Design review of the part built by this model. Coordinates are the model's own, in mm. A direction names the side the tool comes from. Give positions to 0.01 mm unless a question says otherwise; leave off trailing zeros. Order: outer loops, then holes, each group sorted by start corner. A loop starts at its lowest first (then second) coordinate and runs counter-clockwise, first axis right, second up. Notation, with made-up numbers: (87, -2) -> (139, -2) arc R27 ccw to (139, 23) -> close; hole circle Ø6 at (71.25, 10.25). An arc over 180 degrees is marked (long way). One line per item, written item: value. Start each with the question number.
1) Consider section B-B (x = 7.5). State the section outline as (y, z) points.
2) Consider section C-C (y = 30). State the section outline as (x, z) points, plus the area to 3 significant figures.
3) The part is to be moulded in two halves that separate along Y. For faces 5 (the face through (43.196, 2.465, -90.789)), 6 (the face through (6.892, 20.099, -20.006)), 7 (the face through (10, 0, -69)), 8 (the face through (2.81, 31.487, 0.195)), say which applies: released by +Y, released by -Y, zero draft, split by the parting line, or undercut.
4) Wall thickness on line 1 along X through (y, z) = (3, -60); line 2 along Y through (x, z) = (26, -57); line 3 along Y through (x, z) = (17.45, 0): over which ranges is each line inside the solid? List them lowest first. Write a range as from..to.
5) Consider section A-A (z = 0). State the section outline as (x, y) points, plus the area to 3 significant figures.
6) Consider section D-D (z = -34). State the section outline as (x, y) points.
7) Tool access review of faces 1 (the face through (45, 2, -85)), 2 (the face through (13.042, 20.065, -20.073)), 3 (the face through (43.289, 2.465, -79.304)), 4 (the face through (13.196, 2.465, -90.789)): name each direction out of +Z, -Z, +X, -X, +Y, -Y from which nothing blocks a thin tool from reaching the whole face with its end or side.
8) For pin 1 (1.5 mm diameter, centred on y = 2.5, z = -71, fed in from +X); pin 2 (6 mm diameter, centred on y = 9.5, z = -34, fed in from +X); pin 3 (4 mm diameter, centred on y = 30, z = 0, fed in from -X), all flat-tipped, find the tip position at first contact; note any pin that passes through.
from build123d import *

# Parameters (mm, degrees)
SKETCH1_R           = 1.5
BOSS_EXTRUDE1_DEPTH = 20
SKETCH2_W           = 8.6
SKETCH2_H           = 36.312939462
CUT_EXTRUDE1_DEPTH  = 20
FILLET2_R           = 5
SKETCH3_R           = 3.05
BOSS_EXTRUDE3_DEPTH = 5
FILLET3_R           = 5
FILLET4_R           = 5


with BuildPart() as part:
    # Sketch1 → Boss-Extrude1 (new body)
    with BuildSketch(Plane(origin=(0, 0, 0), x_dir=(0, 0, -1), z_dir=(1, 0, 0))):
        with BuildLine():
            Line((2.906888371, 35.813776741), (74.534441854, 0))
            Line((74.534441854, 0), (45.465558146, 0))
            Line((45.465558146, 0), (-2.906888371, 24.186223259))
            ThreePointArc((-2.906888371, 24.186223259), (-5.813776741, 32.906888371), (2.906888371, 35.813776741))
        make_face()
        with Locations((0, 30)):
            Circle(SKETCH1_R, mode=Mode.SUBTRACT)
    extrude(amount=BOSS_EXTRUDE1_DEPTH)

    # Sketch2 → Cut-Extrude1 (cut)
    with BuildSketch(Plane(origin=(0, 29.813776741, -14.906888371), x_dir=(1, 0, 0), z_dir=(0, 0.894427190999916, -0.4472135954999577))):
        with Locations((10, -7.492276671)):
            Rectangle(SKETCH2_W, SKETCH2_H)
    extrude(amount=-CUT_EXTRUDE1_DEPTH, mode=Mode.SUBTRACT)

    # Fillet2
    # the kernel refuses this fillet: 5 mm, written as the material it adds along each edge
    with BuildSketch(Plane(origin=(5.7, 25.04460462, -24.445232613), x_dir=(1, 0, 0), z_dir=(0, -0.894427190999916, 0.4472135954999577)), Plane(origin=(14.3, 25.04460462, -24.445232613), x_dir=(0, 0.44721359549995776, 0.894427190999916), z_dir=(0, -0.894427190999916, 0.4472135954999577))) as fillet2_piece_1:
        with BuildLine():
            CenterArc((FILLET2_R, FILLET2_R), FILLET2_R, 180, 90)
            Line((0, FILLET2_R), (0, 0))
            Line((0, 0), (FILLET2_R, 0))
        make_face()
    extrude(amount=13)

    # Sketch3 → Boss-Extrude3 (add)
    with BuildSketch(Plane.XZ):
        with BuildLine():
            Line((-19, -92.5), (-16, -92.5))
            ThreePointArc((-16, -92.5), (-11.757359313, -90.742640687), (-10, -86.5))
            Line((-10, -86.5), (-10, -85))
            Line((-10, -85), (0, -85))
            Line((0, -85), (0, -86.5))
            ThreePointArc((0, -86.5), (1.757359313, -90.742640687), (6, -92.5))
            Line((6, -92.5), (9, -92.5))
            ThreePointArc((9, -92.5), (13.242640687, -90.742640687), (15, -86.5))
            Line((15, -86.5), (15, -85))
            Line((15, -85), (30, -85))
            Line((30, -85), (30, -86.5))
            ThreePointArc((30, -86.5), (31.757359313, -90.742640687), (36, -92.5))
            Line((36, -92.5), (39, -92.5))
            ThreePointArc((39, -92.5), (43.242640687, -90.742640687), (45, -86.5))
            Line((45, -86.5), (45, -83.5))
            ThreePointArc((45, -83.5), (43.242640687, -79.257359313), (39, -77.5))
            Line((39, -77.5), (37.5, -77.5))
            Line((37.5, -77.5), (37.5, -67.5))
            Line((37.5, -67.5), (39, -67.5))
            ThreePointArc((39, -67.5), (43.242640687, -65.742640687), (45, -61.5))
            Line((45, -61.5), (45, -58.5))
            ThreePointArc((45, -58.5), (43.242640687, -54.257359313), (39, -52.5))
            Line((39, -52.5), (37.5, -52.5))
            Line((37.5, -52.5), (-17.5, -52.5))
            Line((-17.5, -52.5), (-19, -52.5))
            ThreePointArc((-19, -52.5), (-23.242640687, -54.257359313), (-25, -58.5))
            Line((-25, -58.5), (-25, -61.5))
            ThreePointArc((-25, -61.5), (-23.242640687, -65.742640687), (-19, -67.5))
            Line((-19, -67.5), (-17.5, -67.5))
            Line((-17.5, -67.5), (-17.5, -77.5))
            Line((-17.5, -77.5), (-19, -77.5))
            ThreePointArc((-19, -77.5), (-23.242640687, -79.257359313), (-25, -83.5))
            Line((-25, -83.5), (-25, -86.5))
            ThreePointArc((-25, -86.5), (-23.242640687, -90.742640687), (-19, -92.5))
        make_face()
        with Locations(Location((-17.5, -85, 0), (0, 0, 270))):
            Circle(SKETCH3_R, mode=Mode.SUBTRACT)
        with Locations(Location((7.5, -85, 0), (0, 0, 270))):
            Circle(SKETCH3_R, mode=Mode.SUBTRACT)
        with Locations(Location((37.5, -85, 0), (0, 0, 270))):
            Circle(SKETCH3_R, mode=Mode.SUBTRACT)
        with Locations(Location((-17.5, -60, 0), (0, 0, 270))):
            Circle(SKETCH3_R, mode=Mode.SUBTRACT)
        with Locations(Location((37.5, -60, 0), (0, 0, 270))):
            Circle(SKETCH3_R, mode=Mode.SUBTRACT)
    extrude(amount=-BOSS_EXTRUDE3_DEPTH)

    # Fillet3
    fillet3_edges = [part.edges().sort_by_distance(p)[0] for p in [
        (10, 5, -64.534441854),
        (20, 5, -58.517220927),
        (0, 5, -58.517220927),
    ]]
    fillet(fillet3_edges, radius=FILLET3_R)

    # Fillet4
    fillet4_edges = [part.edges().sort_by_distance(p)[0] for p in [
        (0, 5, -52.5),
        (20, 5, -52.5),
    ]]
    fillet(fillet4_edges, radius=FILLET4_R)


solid = part.part
Checked values:
1. outline: (0, -92.5) -> (5, -92.5) -> (5, -88.05) -> (0, -88.05) -> close; (0, -81.95) -> (5, -81.95) -> (5, -65.71) arc R5 cw to (5.53, -63.48) -> (25.56, -23.41) -> (13.93, -17.6) -> (0, -45.47) -> close
2. outline: (0, -14.53) -> (5.7, -14.53) -> (5.7, -1.5) -> (0, -1.5) -> close; (0, 1.5) -> (5.7, 1.5) -> (5.7, 6.5) -> (0, 6.5) -> close; (14.3, -14.53) -> (20, -14.53) -> (20, -1.5) -> (14.3, -1.5) -> close; (14.3, 1.5) -> (20, 1.5) -> (20, 6.5) -> (14.3, 6.5) -> close
2. area: 206 mm^2
3. face 5: zero draft
3. face 6: released by +Y
3. face 7: released by -Y
3. face 8: undercut
4. line 1: x = -25..-20.55, -14.45..34.45, 40.55..45
4. line 2: y = 0..5
4. line 3: y = 22.73..28.5, 31.5..36.5
5. outline: (0, 22.73) -> (5.7, 22.73) -> (5.7, 28.5) -> (0, 28.5) -> close; (0, 31.5) -> (5.7, 31.5) -> (5.7, 36.5) -> (0, 36.5) -> close; (14.3, 22.73) -> (20, 22.73) -> (20, 28.5) -> (14.3, 28.5) -> close; (14.3, 31.5) -> (20, 31.5) -> (20, 36.5) -> (14.3, 36.5) -> close
5. area: 123 mm^2
6. outline: (0, 5.73) -> (20, 5.73) -> (20, 20.27) -> (0, 20.27) -> close
7. face 1: +Z, -Z, +X, +Y, -Y
7. face 2: +Z, +Y
7. face 3: +X, +Y, -Y
7. face 4: -Z, +Y, -Y
8. pin 1: stops at x = 37.5
8. pin 2: stops at x = 20
8. pin 3: stops at x = 0
